The model under review builds one solid part; all positions refer to its coordinate system, in mm. Face numbers are marked on the shaded views. A direction names the side the tool comes from. Give positions to 0.01 mm unless a question says otherwise; leave off trailing zeros. Loops run counter-clockwise (first coordinate to the right, second up) from the corner with the lowest first, then second, coordinate; pieces in that order, holes last. Notation, with made-up numbers: (10.25, 81) - (57.25, 81) arc R32 ccw to (57.25, 110) - close; hole circle Ø10 at (56, -25.5). An arc over 180 degrees is marked (long way). Answer as a JSON object with one key per item and string values.
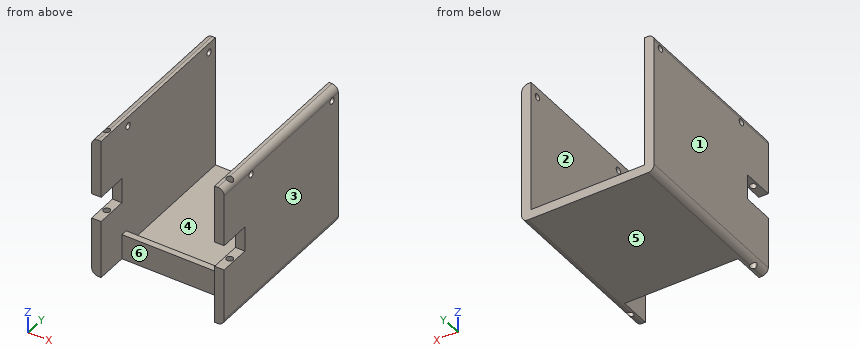
from build123d import *

# Parameters (mm, degrees)
EXTRUDE_1_DEPTH      = 40
EXTRUDE_1_DEPTH_BACK = 5
SKETCH_2_W           = 36
SKETCH_2_H           = 37
CUT_EXTRUDE_1_DEPTH  = 50
SKETCH_5_W           = 36
SKETCH_5_H           = 5
CUT_EXTRUDE_4_DEPTH  = 43
SKETCH_9_R           = 1.025
CUT_EXTRUDE_5_DEPTH  = 45.5
SKETCH_11_W          = 3
SKETCH_11_H          = 18.5
EXTRUDE_5_DEPTH      = 10
SKETCH_13_R          = 1.05
CUT_EXTRUDE_7_DEPTH  = 63.5
FILLET_4_R           = 2
FILLET_5_R           = 2
FILLET_6_R           = 2
FILLET_7_R           = 2


with BuildPart() as part:
    # 草圖1 → 填料-伸長1 (new, two sides: drawn at the far end of the back side and taken through both)
    with BuildSketch(Plane.XY.offset(-EXTRUDE_1_DEPTH_BACK)):
        Polygon((-14.545454545, -28.090909091), (-15.545454545, -28.090909091), (-15.545454545, 16.909090909), (-14.545454545, 16.909090909), (25.454545455, 16.909090909), (26.454545455, 16.909090909), (26.454545455, -28.090909091), (25.454545455, -28.090909091), align=None)
    extrude(amount=EXTRUDE_1_DEPTH + EXTRUDE_1_DEPTH_BACK)

    # 草圖2 → 除料-伸長1 (cut)
    with BuildSketch(Plane(origin=(0, 16.909090909, 0), x_dir=(1, 0, 0), z_dir=(0, 1, 0))):
        with Locations((5.454545455, -21.5)):
            Rectangle(SKETCH_2_W, SKETCH_2_H)
    extrude(amount=-CUT_EXTRUDE_1_DEPTH, mode=Mode.SUBTRACT)

    # 草圖5 → 除料-伸長4 (cut)
    with BuildSketch(Plane(origin=(0, 16.909090909, 0), x_dir=(1, 0, 0), z_dir=(0, 1, 0))):
        with Locations((5.454545455, -0.5)):
            Rectangle(SKETCH_5_W, SKETCH_5_H)
    extrude(amount=-CUT_EXTRUDE_4_DEPTH, mode=Mode.SUBTRACT)

    # 草圖9 → 除料-伸長5 (cut)
    with BuildSketch(Plane.ZY.offset(15.545454545)):
        with Locations(Location((37, -25.090909091, 0), (0, 0, 180))):
            Circle(SKETCH_9_R)
        with Locations(Location((37, 13.909090909, 0), (0, 0, 180))):
            Circle(SKETCH_9_R)
    extrude(amount=-CUT_EXTRUDE_5_DEPTH, mode=Mode.SUBTRACT)

    # 草圖11 → 填料-伸長5 (add)
    with BuildSketch(Plane(origin=(0, -28.090909091, 0), x_dir=(-1, 0, 0), z_dir=(0, -1, 0))):
        with Locations((-24.954545455, -30.75)):
            Rectangle(SKETCH_11_W, SKETCH_11_H)
        with Locations((-24.954545455, -4.25)):
            Rectangle(SKETCH_11_W, SKETCH_11_H)
        with Locations((14.045454545, -30.75)):
            Rectangle(SKETCH_11_W, SKETCH_11_H)
        with Locations((14.045454545, -4.25)):
            Rectangle(SKETCH_11_W, SKETCH_11_H)
    extrude(amount=EXTRUDE_5_DEPTH)

    # 草圖13 → 除料-伸長7 (cut)
    with BuildSketch(Plane(origin=(0, 0, -5), x_dir=(-1, 0, 0), z_dir=(0, 0, -1))):
        with Locations((-24.954545455, -33.090909091)):
            Circle(SKETCH_13_R)
        with Locations((14.045454545, -33.090909091)):
            Circle(SKETCH_13_R)
    extrude(amount=-CUT_EXTRUDE_7_DEPTH, mode=Mode.SUBTRACT)

    # 圓角4
    # the kernel refuses this fillet: 2 mm, written as the material it takes off along each edge
    with BuildSketch(Plane(origin=(26.454545455, 21.909090909, -5), x_dir=(-1, 0, 0), z_dir=(0, -1, 0))) as fillet_4_piece_1:
        with BuildLine():
            CenterArc((FILLET_4_R, -FILLET_4_R), FILLET_4_R, 90, 90)
            Line((0, -FILLET_4_R), (0, 0))
            Line((0, 0), (FILLET_4_R, 0))
        make_face()
    extrude(amount=65, mode=Mode.SUBTRACT)

    # 圓角5
    # the kernel refuses this fillet: 2 mm, written as the material it takes off along each edge
    with BuildSketch(Plane(origin=(-15.545454545, 21.909090909, -5), x_dir=(0, 0, 1), z_dir=(0, -1, 0))) as fillet_5_piece_1:
        with BuildLine():
            CenterArc((FILLET_5_R, -FILLET_5_R), FILLET_5_R, 90, 90)
            Line((0, -FILLET_5_R), (0, 0))
            Line((0, 0), (FILLET_5_R, 0))
        make_face()
    extrude(amount=65, mode=Mode.SUBTRACT)

    # 圓角6
    # the kernel refuses this fillet: 2 mm, written as the material it takes off along each edge
    with BuildSketch(Plane(origin=(26.454545455, -43.090909091, 40), x_dir=(0, 0, -1), z_dir=(0, 1, 0))) as fillet_6_piece_1:
        with BuildLine():
            CenterArc((FILLET_6_R, FILLET_6_R), FILLET_6_R, 180, 90)
            Line((0, FILLET_6_R), (0, 0))
            Line((0, 0), (FILLET_6_R, 0))
        make_face()
    extrude(amount=65, mode=Mode.SUBTRACT)

    # 圓角7
    # the kernel refuses this fillet: 2 mm, written as the material it takes off along each edge
    with BuildSketch(Plane(origin=(-15.545454545, -43.090909091, 40), x_dir=(0, 0, -1), z_dir=(0, 1, 0))) as fillet_7_piece_1:
        with BuildLine():
            CenterArc((FILLET_7_R, -FILLET_7_R), FILLET_7_R, 90, 90)
            Line((0, -FILLET_7_R), (0, 0))
            Line((0, 0), (FILLET_7_R, 0))
        make_face()
    extrude(amount=65, mode=Mode.SUBTRACT)


solid = part.part
Q1. Clearance check with flat-ended pins moving along their axes: pin 1 Ø1.2 at (y, z) = (-25.09, 37) entering from +X; pin 2 Ø9 at (x, z) = (-0.5, -3) entering from -Y; pin 3 Ø2.5 at (x, y) = (-15, -31.5) entering from +Z; pin 4 Ø8 at (x, y) = (0, -7.5) entering from +Z. State where each tip first meets the part, or that it passes through.
Results:
{"pin 1": "passes through", "pin 2": "stops at y = -28.09", "pin 3": "stops at z = 39.99", "pin 4": "stops at z = -2"}
Q2. To check wall thickness, follow probe 1 along X at (y, z) = (0, 36); probe 2 along Z at (x, y) = (8, -14); probe 3 along Y at (x, z) = (25.4, 37). State the ranges of each line that lie inside material, in increasing order. Write a range as [from, to].
Results:
{"probe 1": "x = [-15.55, -12.55], [23.45, 26.45]", "probe 2": "z = [-5, -2]", "probe 3": "y = [-38.09, -34.04], [-32.14, -26.12], [-24.07, 12.88], [14.93, 16.91]"}
Q3. The part is to be moulded in two halves that separate along X. For the marked faces 1, 2 and 3, say which applies: +X half, -X half, draft (parallel to the pull), parting line (faces both ways), or undercut.
Results:
{"face 1": "-X half", "face 2": "undercut", "face 3": "+X half"}
Q4. For the marked faces 4, 5 and 6, list the 3-axis set-ups (+Z, -Z, +X, -X, +Y, -Y) from which the entire face can be reached by the end or side of a thin tool; tool diameter is ignored.
Results:
{"face 4": "+Z, +Y", "face 5": "-Z, +X, -X, +Y, -Y", "face 6": "+Z, -Z, -Y"}
Q5. Consider section C-C, the plane y = -17. State the section outline as (x, z) points, plus the area to 3 significant figures.
Results:
{"outline": "(-15.55, -3) arc R2 ccw to (-13.55, -5) - (24.45, -5) arc R2 ccw to (26.45, -3) - (26.45, 38) arc R2 ccw to (24.45, 40) - (23.45, 40) - (23.45, -2) - (-12.55, -2) - (-12.55, 40) - (-13.55, 40) arc R2 ccw to (-15.55, 38) - close", "area": "375 mm^2"}
Q6. Consider section D-D, the plane x = 1.5. State the section outline as (y, z) points, plus the area to 3 significant figures.
Results:
{"outline": "(-28.09, -5) - (16.91, -5) - (16.91, -2) - (-26.09, -2) - (-26.09, 3) - (-28.09, 3) - close", "area": "145 mm^2"}
Q7. Consider section B-B, the plane z = 37. State the section outline as (x, y) points, plus the area to 3 significant figures.
Results:
{"outline": "(-15.55, -38.09) - (-12.55, -38.09) - (-12.55, -26.12) - (-15.55, -26.12) - close; (-15.55, -24.07) - (-12.55, -24.07) - (-12.55, 12.88) - (-15.55, 12.88) - close; (-15.55, 14.93) - (-12.55, 14.93) - (-12.55, 16.91) - (-15.55, 16.91) - close; (23.45, -38.09) - (26.45, -38.09) - (26.45, -26.12) - (23.45, -26.12) - close; (23.45, -24.07) - (26.45, -24.07) - (26.45, 12.88) - (23.45, 12.88) - close; (23.45, 14.93) - (26.45, 14.93) - (26.45, 16.91) - (23.45, 16.91) - close; hole circle Ø2.1 at (-14.05, -33.09); hole circle Ø2.1 at (24.95, -33.09)", "area": "298 mm^2"}
Q8. Consider section A-A, the plane z = 18. State the section outline as (x, y) points, plus the area to 3 significant figures.
Results:
{"outline": "(-15.55, -28.09) - (-12.55, -28.09) - (-12.55, 16.91) - (-15.55, 16.91) - close; (23.45, -28.09) - (26.45, -28.09) - (26.45, 16.91) - (23.45, 16.91) - close", "area": "270 mm^2"}
